Input: part model. Units: mm. Frame: model coordinates. Face numbers are marked on the shaded views. Coordinates: 2 decimals unless noted, no trailing zeros.
1) Draft query along Y for the marked faces 1, 2, 3 and 4. Return one class per face: pulls with the +Y half, pulls with the -Y half, needs draft (parallel to the pull), parting line crosses it, or undercut.
2) Section query A-A (x = -12). State how many separate pieces and enclosed holes the cut face has, then the cut area to 3 significant figures.
3) Pin query (flat end, axial travel): pin 1 Ø1.5 at (y, z) = (24.5, 10.5) entering from -X; pin 2 Ø4 at (y, z) = (19, -2.5) entering from +X; pin 3 Ø10 at (x, y) = (-14, -7.5) entering from +Z; pin 4 Ø10 at (y, z) = (29, 23) entering from +X. Return the tip coordinate at first contact, or that it passes through.
4) Line query: L1, parallel to Y at x = 5, z = 10; L2, parallel to Y at x = -9, z = -12; L3, parallel to Y at x = -6.5, z = -19.5. Output: solid intervals per line, ascending.
from build123d import *

# Parameters (mm, degrees)
F2_R = 5.08
F3_R = 5.08
F5_R = 20.32
F6_R = 5.08


# Not quite as in the source:
# - a fillet or chamfer that OpenCascade refuses, or shapes differently, is made with other operations: its cross-section is extruded or revolved along the edge and cut away or added


with BuildPart() as f1:
    # F0 (on Top) → F1 (revolve)
    with BuildSketch(Plane.XY):
        with BuildLine():
            Line((0, 41.5879301727), (0, -37.8464572132))
            Line((0, -37.8464572132), (22.0171399415, -37.8464572132))
            Line((22.0171399415, -37.8464572132), (22.0171399415, -31.2269236892))
            Line((22.0171399415, -31.2269236892), (6.7634354346, -26.3342279941))
            Line((6.7634354346, -26.3342279941), (6.7634354346, -11.3683268428))
            ThreePointArc((6.7634354346, -11.3683268428), (14.9158734859, 11.3683268428), (6.7634354346, 34.1049805284))
            Line((6.7634354346, 34.1049805284), (31.2269218266, 41.5879301727))
            Line((31.2269218266, 41.5879301727), (0, 41.5879301727))
        make_face()
    revolve(axis=Axis((0, 1.8707364798, 0), (0, -1, 0)))

    # F2
    f2_edges = [f1.edges().sort_by_distance(p)[0] for p in [
        (-22.01714, -31.226924, 0),
    ]]
    fillet(f2_edges, radius=F2_R)

    # F3
    f3_edges = [f1.edges().sort_by_distance(p)[0] for p in [
        (-6.763435, 34.104981, 0),
    ]]
    fillet(f3_edges, radius=F3_R)

    # F4: fillet of radius 5.08 on 1 edges, made by hand

    # F4_s1 → F4_t2 (revolve, cut)
    with BuildSketch(Plane.XY):
        with BuildLine():
            ThreePointArc((22.0171343212, -34.9324180223), (20.1426258452, -37.0565318577), (17.4220267302, -37.8464572132))
            Line((17.4220267302, -37.8464572132), (22.0171399415, -37.8464572132))
            Line((22.0171399415, -37.8464572132), (22.0171343212, -34.9324180223))
        make_face()
    revolve(axis=Axis((0, -37.8464572132, 0), (0, -1, 0)), mode=Mode.SUBTRACT)

    # F5
    f5_edges = [f1.edges().sort_by_distance(p)[0] for p in [
        (-6.763435, -11.368327, 0),
    ]]
    fillet(f5_edges, radius=F5_R)

    # F6
    f6_edges = [f1.edges().sort_by_distance(p)[0] for p in [
        (-6.763435, -26.334228, 0),
    ]]
    fillet(f6_edges, radius=F6_R)


solid = f1.part
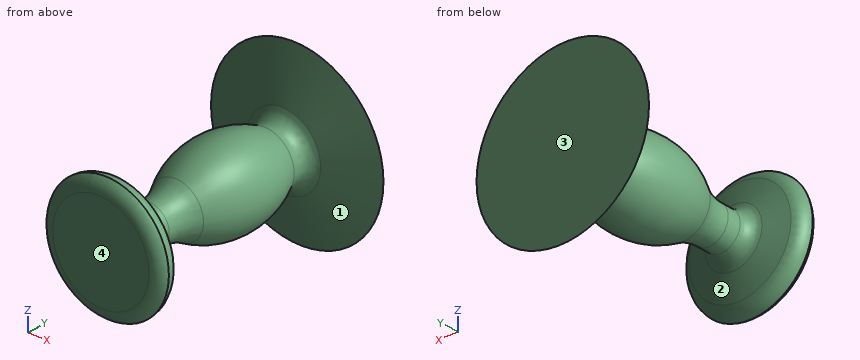
Answer:
1. face 1: undercut
1. face 2: undercut
1. face 3: pulls with the +Y half
1. face 4: pulls with the -Y half
2. separate pieces: 3
2. enclosed holes: 0
2. area: 899 mm2
3. pin 1: stops at x = -7.8
3. pin 2: stops at x = 14.35
3. pin 3: stops at z = 5.14
3. pin 4: passes through
4. L1: y = -37.85 to -27.75, -4.55 to 27.29, 34.8 to 41.59
4. L2: y = -37.85 to -28.98, 36.62 to 41.59
4. L3: y = -36.77 to -31.37, 38.32 to 41.59
